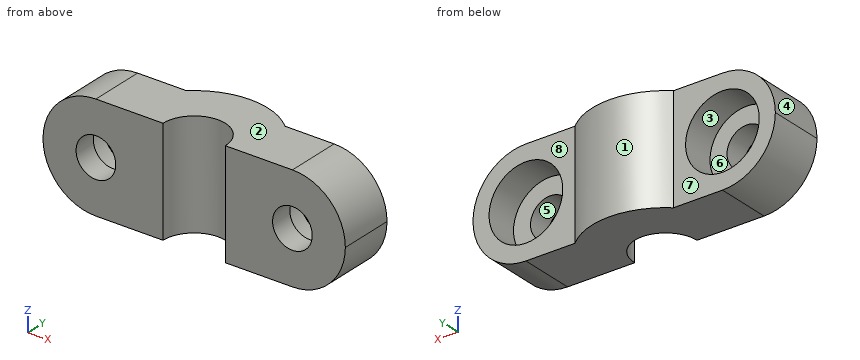
from build123d import *

# Parameters (mm, degrees)
SKETCH1_W           = 40
SKETCH1_H           = 14
BOSS_EXTRUDE1_DEPTH = 7.25
FILLET1_R           = 7
SKETCH2_R           = 2.625
CUT_EXTRUDE1_DEPTH  = 23.395591084
SKETCH3_R           = 4.875
CUT_EXTRUDE2_DEPTH  = 4.25
BOSS_EXTRUDE2_DEPTH = 14
SKETCH5_R           = 4.125
CUT_EXTRUDE3_DEPTH  = 27.288067635


with BuildPart() as part:
    # Sketch1 → Boss-Extrude1 (new body)
    with BuildSketch(Plane(origin=(0, 0, 0), x_dir=(1, 0, 0), z_dir=(0, 1, 0))):
        Rectangle(SKETCH1_W, SKETCH1_H)
    extrude(amount=BOSS_EXTRUDE1_DEPTH)

    # Fillet1
    fillet1_edges = [part.edges().sort_by_distance(p)[0] for p in [
        (-20, 3.625, 7),
        (20, 3.625, 7),
        (20, 3.625, -7),
        (-20, 3.625, -7),
    ]]
    fillet(fillet1_edges, radius=FILLET1_R - 0.0001)  # a hair under: the kernel refuses the full size

    # Sketch2 → Cut-Extrude1 (cut, through all)
    with BuildSketch(Plane(origin=(0, 7.25, 0), x_dir=(1, 0, 0), z_dir=(0, 1, 0))):
        with Locations(Location((-13, 0, 0), (0, 0, 270))):
            Circle(SKETCH2_R)
        with Locations(Location((13, 0, 0), (0, 0, 270))):
            Circle(SKETCH2_R)
    extrude(amount=-CUT_EXTRUDE1_DEPTH, mode=Mode.SUBTRACT)

    # Sketch3 → Cut-Extrude2 (cut)
    with BuildSketch(Plane(origin=(0, 7.25, 0), x_dir=(1, 0, 0), z_dir=(0, 1, 0))):
        with Locations(Location((-13, 0, 0), (0, 0, 270))):
            Circle(SKETCH3_R)
        with Locations(Location((13, 0, 0), (0, 0, 90))):
            Circle(SKETCH3_R)
    extrude(amount=-CUT_EXTRUDE2_DEPTH, mode=Mode.SUBTRACT)

    # Sketch4 → Boss-Extrude2 (add)
    with BuildSketch(Plane.XY.offset(7)):
        with BuildLine():
            Line((6.519202405, 7.25), (-6.519202405, 7.25))
            ThreePointArc((-6.519202405, 7.25), (0, 9.75), (6.519202405, 7.25))
        make_face()
    extrude(amount=-BOSS_EXTRUDE2_DEPTH)

    # Sketch5 → Cut-Extrude3 (cut, through all)
    with BuildSketch(Plane.XY.offset(7)):
        Circle(SKETCH5_R)
    extrude(amount=-CUT_EXTRUDE3_DEPTH, mode=Mode.SUBTRACT)


solid = part.part
Model file for the job. Use its own axes, mm. Face numbers are marked on the shaded views. A direction names the side the tool comes from. Give positions to 0.01 mm unless a question says otherwise; leave off trailing zeros. Loops run counter-clockwise (first coordinate to the right, second up) from the corner with the lowest first, then second, coordinate; pieces in that order, holes last.
1) Saw through at A-A (y = 4.5). Count the separate pieces of the cut face and the enclosed holes in it, plus the area to 3 significant figures.
2) Pull direction Z, two halves, no side cores. Call the marked faces 1, 2 and 3: +Z half, -Z half, draft (parallel to the pull), parting line (faces both ways), or undercut.
3) Flat gauge pins, fed straight in: pin 1 Ø4 at (x, z) = (11.5, -0.5) entering from +Y; pin 2 Ø3 at (x, z) = (13, 0) entering from -Y; pin 3 Ø1.5 at (x, z) = (-1, 2.5) entering from -Y; pin 4 Ø2 at (y, z) = (7, 3) entering from -X. Where does each tip first touch, or does it go through?
4) Tool access for the marked faces 4, 5, 6, 7 and 8: list every direction of +Z, -Z, +X, -X, +Y, -Y with a clear straight run to the whole face (end or side of a thin tool).
5) Saw through at C-C (z = -4.25). Write the cut outline in (x, y) (3 decimals).
6) Saw through at B-B (x = 0). Write the cut outline in (y, z) (3 decimals), plus the area to 4 significant figures.
7) Wall check: line 1 (X direction, y = 5.35, z = 0) (3 decimals); line 2 (X direction, y = 1.25, z = 0) (3 decimals); line 3 (X direction, y = 3.5, z = -1). Give the ranges that are in metal, low to high.
Answer block:
1. separate pieces: 1
1. enclosed holes: 2
1. area: 369 mm2
2. face 1: draft
2. face 2: +Z half
2. face 3: undercut
3. pin 1: stops at y = 3
3. pin 2: passes through
3. pin 3: stops at y = 3.74
3. pin 4: stops at x = -19.71
4. face 4: +Z, -X, +Y, -Y
4. face 5: +Y, -Y
4. face 6: +Y
4. face 7: +Z, -Z, -X, +Y
4. face 8: +Z, -Z, +X, +Y
5. outline: (-18.562, 0) - (-4.125, 0) arc R4.125 cw to (4.125, 0) - (18.562, 0) - (18.562, 7.25) - (15.388, 7.25) - (15.388, 3) - (10.612, 3) - (10.612, 7.25) - (6.519, 7.25) arc R9.75 ccw to (-6.519, 7.25) - (-10.612, 7.25) - (-10.612, 3) - (-15.388, 3) - (-15.388, 7.25) - (-18.562, 7.25) - close
6. outline: (4.125, -7) - (9.75, -7) - (9.75, 7) - (4.125, 7) - close
6. area: 78.75 mm2
7. line 1: x = -20 to -17.875, -8.125 to 8.125, 17.875 to 20
7. line 2: x = -20 to -15.625, -10.375 to -3.931, 3.931 to 10.375, 15.625 to 20
7. line 3: x = -19.93 to -17.77, -8.23 to -2.18, 2.18 to 8.23, 17.77 to 19.93
